Design review of the part built by this model. Coordinates are the model's own, in mm. A direction names the side the tool comes from. Coordinates: 2 decimals unless noted, no trailing zeros. Write each loop counter-clockwise with the first axis right and the second up, starting at its lowest first coordinate (ties: lowest second). Pieces come first, ordered by that corner, then holes. Notation, with made-up numbers: M 61.25,-32 L 114.25,-32 A23 cw 114.25,-20 Z; hole C -26,80.25 d6. An arc over 180 degrees is marked long. One line per question, with ' | ' between items.
from build123d import *

# Parameters (mm, degrees)
SKETCH1_W           = 120
SKETCH1_H           = 80
BOSS_EXTRUDE1_DEPTH = 10
SKETCH2_W           = 22.4
SKETCH2_H           = 12.5
CUT_EXTRUDE1_DEPTH  = 10
SKETCH3_W           = 10
SKETCH3_H           = 80
BOSS_EXTRUDE2_DEPTH = 20
SKETCH4_R           = 1
CUT_EXTRUDE3_DEPTH  = 12


with BuildPart() as part:
    # Sketch1 → Boss-Extrude1 (new body)
    with BuildSketch(Plane(origin=(0, 0, 0), x_dir=(1, 0, 0), z_dir=(0, 1, 0))):
        Rectangle(SKETCH1_W, SKETCH1_H)
    extrude(amount=BOSS_EXTRUDE1_DEPTH)

    # Sketch2 → Cut-Extrude1 (cut)
    with BuildSketch(Plane(origin=(0, 10, 0), x_dir=(1, 0, 0), z_dir=(0, 1, 0))):
        with Locations((30, 0)):
            Rectangle(SKETCH2_W, SKETCH2_H)
    extrude(amount=-CUT_EXTRUDE1_DEPTH, mode=Mode.SUBTRACT)

    # Sketch3 → Boss-Extrude2 (add)
    with BuildSketch(Plane.XZ):
        with Locations((-55, 0)):
            Rectangle(SKETCH3_W, SKETCH3_H)
        with Locations((55, 0)):
            Rectangle(SKETCH3_W, SKETCH3_H)
    extrude(amount=BOSS_EXTRUDE2_DEPTH)

    # Sketch4 → Cut-Extrude3 (cut)
    with BuildSketch(Plane(origin=(0, 10, 0), x_dir=(1, 0, 0), z_dir=(0, 1, 0))):
        with Locations(Location((16.15, 0, 0), (0, 0, 270))):
            Circle(SKETCH4_R)
        with Locations(Location((43.85, 0, 0), (0, 0, 270))):
            Circle(SKETCH4_R)
    extrude(amount=-CUT_EXTRUDE3_DEPTH, mode=Mode.SUBTRACT)


solid = part.part
1. Take a section at B-B (y = 7.5). Write out the cut boundary in (x, z), then the cut area to 3 significant figures.
Answer sheet:
outline: M -60,-40 L 60,-40 L 60,40 L -60,40 Z; hole C 16.15,0 d2; hole M 18.8,-6.25 L 41.2,-6.25 L 41.2,6.25 L 18.8,6.25 Z; hole C 43.85,0 d2 | area: 9,310 mm^2
2. Draft analysis for pull direction X (two halves, no side actions). For faces 1 (the face through (-60, -5, -1)), 2 (the face through (-1, 2, -40)), 3 (the face through (-50, -10, -1)), state which applies: pulls with the +X half, pulls with the -X half, needs draft (parallel to the pull), parting line crosses it, or undercut.
Answer sheet:
face 1: pulls with the -X half | face 2: needs draft | face 3: undercut
3. Take a section at D-D (z = -8). Write out the cut boundary in (x, y).
Answer sheet:
outline: M -60,-20 L -50,-20 L -50,0 L 50,0 L 50,-20 L 60,-20 L 60,10 L -60,10 Z
4. Take a section at A-A (x = 30). Write out the cut boundary in (y, z), then the cut area to 3 significant figures.
Answer sheet:
outline: M 0,-40 L 10,-40 L 10,-6.25 L 0,-6.25 Z; M 0,6.25 L 10,6.25 L 10,40 L 0,40 Z | area: 675 mm^2
5. To check wall thickness, follow line 1 along X through (y, z) = (6.5, 0); line 2 along X through (y, z) = (-11, -20); line 3 along Y through (x, z) = (-2, 33). State the ranges of each line that lie inside material, in increasing order. Write a range as [from, to].
Answer sheet:
line 1: [-60, 15.15], [17.15, 18.8], [41.2, 42.85], [44.85, 60] | line 2: [-60, -50], [50, 60] | line 3: [0, 10]
6. Take a section at C-C (z = 3). Write out the cut boundary in (x, y).
Answer sheet:
outline: M -60,-20 L -50,-20 L -50,0 L 18.8,0 L 18.8,10 L -60,10 Z; M 41.2,0 L 50,0 L 50,-20 L 60,-20 L 60,10 L 41.2,10 Z
7. Insertion check: pin 1 Ø24 at (x, z) = (-11.5, 8) entering from -Y. The pin has a flat end and moves straight along its axis. Give the tip position at first contact, or say it passes through.
Answer sheet:
pin 1: y = 0
8. Tool access review of faces 4 (the face through (30, 5, 6.25)), 5 (the face through (-1, 2, 40)), 6 (the face through (50, -10, -1)): name each direction out of +Z, -Z, +X, -X, +Y, -Y from which nothing blocks a thin tool from reaching the whole face with its end or side.
Answer sheet:
face 4: +Y, -Y | face 5: +Z, +X, -X, +Y, -Y | face 6: +Z, -Z, -Y
